Model file for the job. Use its own axes, mm. A direction names the side the tool comes from. Round coordinates to 2 decimals unless told otherwise and drop trailing zeros. Loops run counter-clockwise (first coordinate to the right, second up) from the corner with the lowest first, then second, coordinate; pieces in that order, holes last. Notation, with made-up numbers: M 46.25,-25 L 63.25,-25 A5 cw 63.25,-21 Z; hole C 26,-15 d2. An arc over 180 degrees is marked long. Use a Markdown table: item, result. Add a question column.
Q1. Cut at A-A (y = 3). Give the cut face in (x, z), plus the area to 3 significant figures.
Q2. Tool access for faces 1 (the face through (-50, -1, 12)), 2 (the face through (0, -45, 13)): list every direction of +Z, -Z, +X, -X, +Y, -Y with a clear straight run to the whole face (end or side of a thin tool).
Q3. Cut at B-B (x = 0). Give the cut face in (y, z).
Q4. Probe line 1 (X direction, y = 34, z = 12.5); line 2 (X direction, y = -44, z = 5); line 3 (Y direction, x = 1.5, z = 11.25). List the from-to ranges inside material, lowest first. Write a range as from..to.
Q5. Cut at C-C (z = 6.5). Give the cut face in (x, y).
Q6. Mould opens along Y. For faces 3 (the face through (-12, 1, 0)), 4 (the face through (1, -75, 12)), 5 (the face through (-5, -1, 13)) say: +Y half, -Y half, draft (parallel to the pull), parting line (faces both ways), or undercut.
Autodesk Inventor part; units mm, degrees
ref_plane "YZ Plane" through (0, 0, 0) normal (1, 0, 0) x (0, 1, 0)
ref_plane "XZ Plane" through (0, 0, 0) normal (0, 1, 0) x (-1, 0, 0)
ref_plane "XY Plane" through (0, 0, 0) normal (0, 0, 1) x (1, 0, 0)
sketch "Sketch1" plane through (0, 0, 0) normal (0, 0, 1) x (1, 0, 0)
  line L0 (-50, 75) -> (50, 75)
  line L1 (50, 75) -> (50, -75)
  line L2 (50, -75) -> (-50, -75)
  line L3 (-50, -75) -> (-50, 75)
  point P0 (0, 0)
  point P1 (0, 75)
  point P2 (-50, 0)
  dimension "d0" = 100
  dimension "d1" = 150
extrude "Extrusion1" add sketch "Sketch1" along normal blind 25
sketch "Sketch2" plane through (0, 0, 25) normal (0, 0, 1) x (1, 0, 0)
  line L0 (-50, -75) -> (50, -75)
  line L1 (0, -75) -> (0, -50) construction
  line L2 (0, -50) -> (0, -40) construction
  line L3 (-5, 40) -> (5, 40) construction
  line L4 (5, 40) -> (5, -40)
  line L5 (5, -40) -> (-5, -40) construction
  line L6 (-5, -40) -> (-5, 40)
  arc A0 (-5, -40) -> (5, -40) centre (0, -40) ccw
  arc A1 (5, 40) -> (-5, 40) centre (0, 40) ccw
  line L7 (50, 75) -> (-50, 75)
  line L8 (0, 75) -> (0, 50) construction
  line L9 (0, 50) -> (0, 40) construction
  point P0 (0, 0)
  dimension "d4" = 25
  dimension "d5" = 10
  dimension "d6" = 10
  dimension "d8" = 25
  dimension "d11" = 10
extrude "Extrusion2" cut sketch "Sketch2" against normal through all
properties part number "Foam_Hammer_Side" material "Polystyrene, Expanded"
Checked values:
| question | item | result |
|---|---|---|
| 1 | outline | M -50,0 L -5,0 L -5,25 L -50,25 Z; M 5,0 L 50,0 L 50,25 L 5,25 Z |
| 1 | area | 2,250 mm^2 |
| 2 | face 1 | +Z, -Z, -X, +Y, -Y |
| 2 | face 2 | +Z, -Z |
| 3 | outline | M -75,0 L -45,0 L -45,25 L -75,25 Z; M 45,0 L 75,0 L 75,25 L 45,25 Z |
| 4 | line 1 | x = -50..-5, 5..50 |
| 4 | line 2 | x = -50..-3, 3..50 |
| 4 | line 3 | y = -75..-44.77, 44.77..75 |
| 5 | outline | M -50,-75 L 50,-75 L 50,75 L -50,75 Z; hole M -5,-40 A5 ccw 5,-40 L 5,40 A5 ccw -5,40 Z |
| 6 | face 3 | draft |
| 6 | face 4 | -Y half |
| 6 | face 5 | undercut |
